Read the model definition and answer for the solid it produces. Units are mm, in the model's axes. A direction names the side the tool comes from. Give positions to 0.01 mm unless a question says otherwise; leave off trailing zeros. Write each loop counter-clockwise with the first axis right and the second up, starting at its lowest first coordinate (ties: lowest second). Pieces come first, ordered by that corner, then holes. Notation, with made-up numbers: M 17.5,2 L 64.5,2 A35 cw 64.5,38 Z; hole C 1,-22.75 d8. An arc over 180 degrees is marked long. Write each question's results on one line, items separated by ' | '. Start each with the question number.
```python
from build123d import *

# Parameters (mm, degrees)
SKETCH1_W                    = 1193.8
SKETCH1_H                    = 53.975
BASE_FLANGE1_DEPTH           = 2.58826
EDGE_FLANGE1_STRIP_W         = 13.40104
EDGE_FLANGE1_STRIP_H         = 2.58826
EDGE_FLANGE1_STRIP_CUT_DEPTH = 1193.8
EDGE_FLANGE1_DEPTH           = 1193.8
F_1_4_CLEARANCE_HOLE1_D      = 6.7564


# Sheet-metal steps are written as plain solids
with BuildPart() as part:
    # Sketch1 → Base-Flange1 (new body)
    with BuildSketch(Plane(origin=(0, 0, 0), x_dir=(1, 0, 0), z_dir=(0, 1, 0))):
        Rectangle(SKETCH1_W, SKETCH1_H)
    extrude(amount=-BASE_FLANGE1_DEPTH)

    # Edge-Flange1 strip (across the edge) → Edge-Flange1 strip cut (cut)
    with BuildSketch(Plane(origin=(596.9, -2.58826, 26.9875), x_dir=(0, 0, -1), z_dir=(-1, 0, 0))):
        with Locations((-5.17652, -1.29413)):
            Rectangle(EDGE_FLANGE1_STRIP_W, EDGE_FLANGE1_STRIP_H)
    extrude(amount=EDGE_FLANGE1_STRIP_CUT_DEPTH, mode=Mode.SUBTRACT)

    # Edge-Flange1 section (across the edge) → Edge-Flange1 (add)
    with BuildSketch(Plane(origin=(596.9, -2.58826, 26.9875), x_dir=(0, 0, -1), z_dir=(-1, 0, 0))):
        with BuildLine():
            Line((-2.58826, 1.524), (-2.58826, 50.8))
            Line((-2.58826, 50.8), (0, 50.8))
            Line((0, 50.8), (0, 1.524))
            ThreePointArc((0, 1.524), (0.446369265, 0.446369265), (1.524, 0))
            Line((1.524, 0), (1.524, -2.58826))
            ThreePointArc((1.524, -2.58826), (-1.383806932, -1.383806932), (-2.58826, 1.524))
        make_face()
    extrude(amount=EDGE_FLANGE1_DEPTH)

    # 1/4 Clearance Hole1 (through all)
    with Locations(Plane(origin=(0, 0, 0), x_dir=(1, 0, 0), z_dir=(0, 1, 0))):
        with Locations((565.15, 6.0325), (-565.15, 6.0325)):
            Hole(F_1_4_CLEARANCE_HOLE1_D / 2)


solid = part.part
```
Item 1: Given P1, Ø15, axis at x = 267.5, y = -21.5, coming from the -Z side; P2, Ø4, axis at x = -263, z = -12, coming from the -Y side; P3, Ø6, axis at x = -565.15, z = -6.03, coming from the -Y side, each flat-ended and moving along its own axis, determine where each tip first touches the part or whether it passes through.
Item 2: Section A-A, the plane x = -382 is taken. Determine the outline of the cut face in (y, z), then the cut area to 3 significant figures.
Item 3: Determine the mould class of faces 1 (the flat face through (8, -29, 26.988)), 2 (the flat face through (8, -28, 29.576)), 3 (the flat face through (-8, 0, -1)) for opening direction Z: +Z half, -Z half, draft (parallel to the pull), parting line (faces both ways), or undercut.
Item 4: Section C-C, the plane z = 8.5 is taken. Determine the outline of the cut face in (x, y), then the cut area to 3 significant figures.
Item 5: Straight lines are drawn through the part: line 1 (Z direction, x = 112, y = -21); line 2 (Y direction, x = -404.5, z = -7); line 3 (Z direction, x = 565.15, y = -1.95). For each, find the intervals that lie inside material, in ascending order.
Item 6: For faces 4 (the flat face through (596.9, -1, 14)), 5 (the flat face through (-8, -2.588, -1)), determine the directions among +Z, -Z, +X, -X, +Y, -Y from which every point of the face is accessible in a straight line to the end or side of a thin tool.
Item 7: Section B-B, the plane y = -36 is taken. Determine the outline of the cut face in (x, z), then the cut area to 3 significant figures.
Worked out:
1) P1: stops at z = 26.99 | P2: stops at y = -2.59 | P3: passes through
2) outline: M -53.39,26.99 L -4.11,26.99 A1.52 cw -2.59,25.46 L -2.59,-26.99 L 0,-26.99 L 0,25.46 A4.11 ccw -4.11,29.58 L -53.39,29.58 Z | area: 275 mm²
3) face 1: -Z half | face 2: +Z half | face 3: draft
4) outline: M -596.9,-2.59 L 596.9,-2.59 L 596.9,0 L -596.9,0 Z | area: 3,090 mm²
5) line 1: z = 26.99 to 29.58 | line 2: y = -2.59 to 0 | line 3: z = -26.99 to -9.41, -2.65 to 28.96
6) face 4: +Z, -Z, +X, +Y, -Y | face 5: -Z, +X, -X, -Y
7) outline: M -596.9,26.99 L 596.9,26.99 L 596.9,29.58 L -596.9,29.58 Z | area: 3,090 mm²
